Design review of the part built by this model. Coordinates are the model's own, in mm. A direction names the side the tool comes from. Give positions to 0.01 mm unless a question says otherwise; leave off trailing zeros. Loops run counter-clockwise (first coordinate to the right, second up) from the corner with the lowest first, then second, coordinate; pieces in that order, holes last.
from build123d import *

# Parameters (mm, degrees)
F0_W     = 6
F0_H     = 240
F1_DEPTH = 180
F3_START = -3
F2_W     = 3
F2_H     = 3
F3_DEPTH = 234
F4_W     = 6
F4_H     = 20
F5_DEPTH = 6.001


with BuildPart() as f1:
    # F0 (on Top) → F1 (new body)
    with BuildSketch(Plane.XY):
        Rectangle(F0_W, F0_H)
    extrude(amount=F1_DEPTH)

    # F2 (on face) → F3 (cut)
    with BuildSketch(Plane.XZ.offset(120).offset(F3_START)):
        with Locations((1.5, 11.5)):
            Rectangle(F2_W, F2_H)
    extrude(amount=-F3_DEPTH, mode=Mode.SUBTRACT)

    # F4 (on face) → F5 (cut, through all)
    with BuildSketch(Plane.YZ.offset(3)):
        with Locations((-117, 30)):
            Rectangle(F4_W, F4_H)
        with Locations((-117, 70)):
            Rectangle(F4_W, F4_H)
        with Locations((-117, 110)):
            Rectangle(F4_W, F4_H)
        with Locations((-117, 150)):
            Rectangle(F4_W, F4_H)
        with Locations((117, 150)):
            Rectangle(F4_W, F4_H)
        with Locations((117, 110)):
            Rectangle(F4_W, F4_H)
        with Locations((117, 70)):
            Rectangle(F4_W, F4_H)
        with Locations((117, 30)):
            Rectangle(F4_W, F4_H)
    extrude(amount=-F5_DEPTH, mode=Mode.SUBTRACT)


solid = f1.part
Q1. Take a section at A-A (z = 106.5). Give the boundary of the cut face in (x, y).
Results:
outline: (-3, -114) - (3, -114) - (3, 114) - (-3, 114) - close
Q2. Wall thickness on line 1 (Z direction, x = 2.7, y = -89); line 2 (Y direction, x = 2.05, z = 144): over which ranges is each line inside the solid? List them lowest first.
Results:
line 1: z = 0 to 10, 13 to 180
line 2: y = -114 to 114
Q3. Insertion check: pin 1 (1.8 mm diameter, centred on x = 0, z = 65.5, fed in from -Y). The pin has a flat end and moves straight along its axis. Give the tip position at first contact, or say it passes through.
Results:
pin 1: stops at y = -114
Q4. Draft analysis for pull direction Z (two halves, no side actions). For faces 1 (the face through (0, 117, 140)), 2 (the face through (0, 2, 180)), 3 (the face through (0, 120, 10)), state which applies: pulls with the +Z half, pulls with the -Z half, needs draft (parallel to the pull), parting line crosses it, or undercut.
Results:
face 1: undercut
face 2: pulls with the +Z half
face 3: needs draft
Q5. Tool access review of faces 4 (the face through (0, -120, 10)), 5 (the face through (0, -117, 140)), 6 (the face through (0, 117, 60)): name each direction out of +Z, -Z, +X, -X, +Y, -Y from which nothing blocks a thin tool from reaching the whole face with its end or side.
Results:
face 4: +Z, -Z, +X, -X, -Y
face 5: +X, -X, -Y
face 6: +X, -X, +Y
